The listing builds one solid part. Answer for the finished solid, in the listing's coordinates (mm). Coordinates: 2 decimals unless noted, no trailing zeros. Order: outer loops, then holes, each group sorted by start corner. A loop starts at its lowest first (then second) coordinate and runs counter-clockwise, first axis right, second up. Notation, with made-up numbers: (20.5, 34) -> (30.5, 34) arc R29 cw to (30.5, 63) -> close; hole circle Ø3 at (33, 81). An arc over 180 degrees is marked (long way). One line per question, with ' | ' between items.
from build123d import *

# Parameters (mm, degrees)
SKETCH_1_W      = 12
SKETCH_1_H      = 12
SKETCH_1_W_2    = 7
SKETCH_1_H_2    = 3
SKETCH_1_R      = 1
EXTRUDE_1_DEPTH = 0.4
EXTRUDE_START   = 0.4
SKETCH_1_5_R    = 3.5
EXTRUDE_2_DEPTH = 10.6
SKETCH_1_6_R    = 4
EXTRUDE_3_DEPTH = 0.01
FILLET_1_R      = 1.5


with BuildPart() as part:
    # 草图1 → 凸台-拉伸1 (new body)
    # profile 1 of 2: a face of its own
    with BuildSketch(Plane(origin=(0, 0, 0), x_dir=(1, 0, 0), z_dir=(0, 1, 0))):
        Rectangle(SKETCH_1_W, SKETCH_1_H)
    # profile 2 of 2: a face of its own
    with BuildSketch(Plane(origin=(0, 0, 0), x_dir=(1, 0, 0), z_dir=(0, 1, 0))):
        with Locations((-9.5, 0)):
            Rectangle(SKETCH_1_W_2, SKETCH_1_H_2)
        with Locations(Location((-11.5, 0, 0), (0, 0, 270))):
            Circle(SKETCH_1_R, mode=Mode.SUBTRACT)
    extrude(amount=EXTRUDE_1_DEPTH)

    # 草图1<5> → 凸台-拉伸2 (add)
    with BuildSketch(Plane(origin=(0, 0, 0), x_dir=(1, 0, 0), z_dir=(0, 1, 0)).offset(EXTRUDE_START)):
        with Locations(Location((0, 0, 0), (0, 0, 90))):
            Circle(SKETCH_1_5_R)
    extrude(amount=EXTRUDE_2_DEPTH)

    # 草图1<6> → 凸台-拉伸3 (add)
    with BuildSketch(Plane(origin=(0, 0, 0), x_dir=(1, 0, 0), z_dir=(0, 1, 0)).offset(EXTRUDE_START)):
        with Locations(Location((0, 0, 0), (0, 0, 90))):
            Circle(SKETCH_1_6_R)
    extrude(amount=EXTRUDE_3_DEPTH)

    # loft up to a face of the part (loft_1)
    loft([Face(Wire([part.edges().sort_by_distance((-2.551390196, 11, 2.395914871))[0]])), Face(Wire([part.edges().sort_by_distance((-2.91587451, 0.4, 2.738188424))[0]]))])

    # 圆角1
    fillet_1_edges = [part.edges().sort_by_distance(p)[0] for p in [
        (-13, 0.2, 1.5),
        (-13, 0.2, -1.5),
    ]]
    fillet(fillet_1_edges, radius=FILLET_1_R - 0.0001)  # a hair under: the kernel refuses the full size


solid = part.part
Item 1: Section A-A, the plane x = -4.75 is taken. Give the vertices of the cut face in (y, z), plus the area to 3 significant figures.
Computed values:
outline: (0, -6) -> (0.4, -6) -> (0.4, 6) -> (0, 6) -> close | area: 4.80 mm^2
Item 2: Section C-C, the plane y = 7.5 is taken. Give the vertices of the cut face in (x, z), plus the area to 3 significant figures.
Computed values:
outline: circle Ø7.33 at (0, 0) | area: 42.2 mm^2
Item 3: Section D-D, the plane y = 2.25 is taken. Give the vertices of the cut face in (x, z), plus the area to 3 significant figures.
Computed values:
outline: circle Ø7.83 at (0, 0) | area: 48.1 mm^2
Item 4: Determine the mould class of faces 1 (the face through (-10.51, 0.2, -0.13)), 2 (the face through (-12.57, 0.2, -1.05)), 3 (the face through (-4, 0.4, -3)) for opening direction X: pulls with the +X half, pulls with the -X half, needs draft (parallel to the pull), parting line crosses it, or undercut.
Computed values:
face 1: undercut | face 2: pulls with the -X half | face 3: needs draft
Item 5: Each of these flat-tipped pins is pushed along its axis until it touches: pin 1 Ø4 at (x, y) = (3.5, 4) entering from -Z; pin 2 Ø6 at (x, y) = (2, 7) entering from +Z; pin 3 Ø4 at (x, y) = (-3, 4) entering from -Z; pin 4 Ø2 at (x, z) = (-2.5, -4) entering from -Y. Where does it stop, or does it pass through?
Computed values:
pin 1: stops at z = -3.53 | pin 2: stops at z = 3.8 | pin 3: stops at z = -3.71 | pin 4: stops at y = 0
Item 6: Find the intervals of material crossed by L1, parallel to X at y = 0.2, z = 0; L2, parallel to Y at x = 3.25, z = 5.25; L3, parallel to X at y = 4, z = -3.25, in increasing order.
Computed values:
L1: x = -13 to -12.5, -10.5 to 6 | L2: y = 0 to 0.4 | L3: x = -2.03 to 2.03
Item 7: Section B-B, the plane z = -5 is taken. Give the vertices of the cut face in (x, y), plus the area to 3 significant figures.
Computed values:
outline: (-6, 0) -> (6, 0) -> (6, 0.4) -> (-6, 0.4) -> close | area: 4.80 mm^2
